from build123d import *

# Parameters (mm, degrees)
SKETCH_1_R                      = 12.55
EXTRUDE_1_DEPTH                 = 6
SKETCH_2_R                      = 3.2
CUT_EXTRUDE_1_DEPTH             = 6
CUT_EXTRUDE_2_REACH             = 20.735
SKETCH_3_R                      = 1
CUT_EXTRUDE_2_DIRECTION_2_REACH = 20.735
SKETCH_4_R                      = 13.5
EXTRUDE_2_DEPTH                 = 5
SKETCH_5_R                      = 12.5
CUT_EXTRUDE_3_DEPTH             = 5
FILLET_2_R                      = 2


with BuildPart() as part:
    # 草图1 → 凸台-拉伸1 (new body)
    with BuildSketch(Plane(origin=(0, 0, 0), x_dir=(0, 0, -1), z_dir=(1, 0, 0))):
        Circle(SKETCH_1_R)
    extrude(amount=EXTRUDE_1_DEPTH)

    # 草图2 → 切除-拉伸1 (cut)
    with BuildSketch(Plane.ZY):
        Circle(SKETCH_2_R)
    extrude(amount=-CUT_EXTRUDE_1_DEPTH, mode=Mode.SUBTRACT)

    # 草图3 → 切除-拉伸2 (cut, up to next)
    with BuildSketch(Plane(origin=(0, 0, 0), x_dir=(1, 0, 0), z_dir=(0, 1, 0)), mode=Mode.PRIVATE) as cut_extrude_2_sk1:
        with Locations(Location((3, 0, 0), (0, 0, 270))):
            Circle(SKETCH_3_R)
    cut_extrude_2_tool1 = extrude(cut_extrude_2_sk1.sketch, amount=-CUT_EXTRUDE_2_REACH, mode=Mode.PRIVATE) & part.part
    add(cut_extrude_2_tool1.solids().sort_by_distance((3, 0, 0))[0], mode=Mode.SUBTRACT)

    # 草图3 → 切除-拉伸2 direction 2 (cut, up to next)
    with BuildSketch(Plane(origin=(0, 0, 0), x_dir=(1, 0, 0), z_dir=(0, 1, 0)), mode=Mode.PRIVATE) as cut_extrude_2_direction_2_sk1:
        with Locations(Location((3, 0, 0), (0, 0, 270))):
            Circle(SKETCH_3_R)
    cut_extrude_2_direction_2_tool1 = extrude(cut_extrude_2_direction_2_sk1.sketch, amount=CUT_EXTRUDE_2_DIRECTION_2_REACH, mode=Mode.PRIVATE) & part.part
    add(cut_extrude_2_direction_2_tool1.solids().sort_by_distance((3, 0, 0))[0], mode=Mode.SUBTRACT)

    # 草图4 → 凸台-拉伸2 (add)
    with BuildSketch(Plane(origin=(6, 0, 0), x_dir=(0, 0, -1), z_dir=(1, 0, 0))):
        Circle(SKETCH_4_R)
    extrude(amount=EXTRUDE_2_DEPTH)

    # 草图5 → 切除-拉伸3 (cut)
    with BuildSketch(Plane(origin=(11, 0, 0), x_dir=(0, 0, -1), z_dir=(1, 0, 0))):
        Circle(SKETCH_5_R)
    extrude(amount=-CUT_EXTRUDE_3_DEPTH, mode=Mode.SUBTRACT)

    # 圆角2
    # the kernel refuses this fillet: 2 mm, written as the material it adds along each edge
    with BuildSketch(Plane(origin=(6, 0, 0), x_dir=(0, 0, -1), z_dir=(0, -1, 0))) as fillet_2_piece_1:
        with BuildLine():
            CenterArc((14.55, -1.702204453), FILLET_2_R, 121.668243254, 58.331756746)
            Line((12.55, -1.702204453), (12.51, -1.702204453))
            Line((12.51, -1.702204453), (12.51, 0))
            Line((12.51, 0), (12.55, 0.04))
            ThreePointArc((12.55, 0.04), (13.025, 0.04), (13.479, 0.034044089))
            Line((13.479, 0.034044089), (13.5, 0))
        make_face()
    revolve(axis=Axis((6, 0, 0), (1, 0, 0)))


solid = part.part
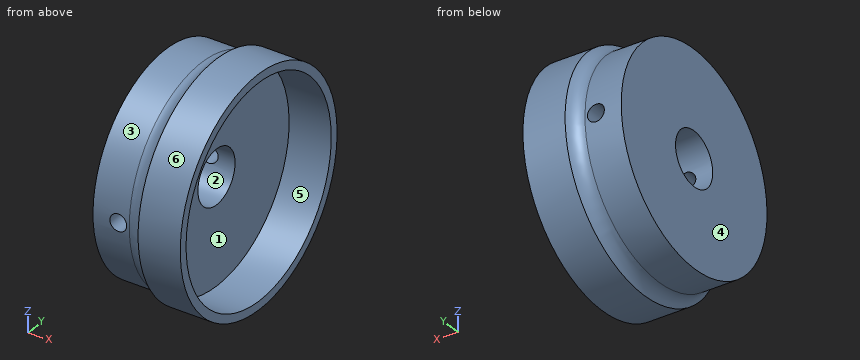
Design review of the part built by this model. Coordinates are the model's own, in mm. Face numbers are marked on the shaded views. A direction names the side the tool comes from. Give positions to 0.01 mm unless a question says otherwise; leave off trailing zeros. Order: outer loops, then holes, each group sorted by start corner. A loop starts at its lowest first (then second) coordinate and runs counter-clockwise, first axis right, second up. Notation, with made-up numbers: (16, 30.5) - (68, 30.5) arc R19 cw to (68, 53.5) - close; hole circle Ø1 at (48.25, 71.5). An arc over 180 degrees is marked (long way). Write item = value, one per line. Start each with the question number.
Q1. Tool access review of the marked faces 1, 2 and 3: name each direction out of +Z, -Z, +X, -X, +Y, -Y from which nothing blocks a thin tool from reaching the whole face with its end or side.
Q2. We need section A-A on y = 0. State the section outline as (x, z) points, plus the area to 3 significant figures.
Q3. We need section C-C on x = 3. State the section outline as (y, z) points.
Q4. We need section B-B on z = 0. State the section outline as (x, y) points.
Q5. To check wall thickness, follow L1, parallel to X at y = 7.75, z = 0; L2, parallel to X at y = 8, z = 6.5; L3, parallel to Y at x = 9.75, z = 9.75. State the ranges of each line that lie inside material, in increasing order. Write a range as from..to.
Q6. We need section D-D on x = 6.5. State the section outline as (y, z) points.
Q7. Clearance check with flat-ended pins moving along their axes: pin 1 Ø6 at (y, z) = (0, 0) entering from +X; pin 2 Ø3 at (x, z) = (2.5, -9) entering from -Y; pin 3 Ø2 at (x, z) = (2.5, -0.5) entering from +Y; pin 4 Ø3 at (x, z) = (3, 0) entering from +Y. State where each tip first meets the part, or that it passes through.
Q8. Mouldability with a two-part tool opening along Y and no side actions: class the marked faces 4, 5 and 6 as released by +Y, released by -Y, zero draft, split by the parting line, or undercut.
Working result:
q1.face_1 = +X
q1.face_2 = +X, -X
q1.face_3 = -X
q2.outline = (0, -12.55) - (4.3, -12.55) arc R2 cw to (6, -13.5) - (11, -13.5) - (11, -12.5) - (6, -12.5) - (6, -3.2) - (0, -3.2) - close; (0, 3.2) - (6, 3.2) - (6, 12.5) - (11, 12.5) - (11, 13.5) - (6, 13.5) arc R2 cw to (4.3, 12.55) - (0, 12.55) - close
q2.area = 123 mm²
q3.outline = (-12.51, -1) arc R12.55 ccw to (12.51, -1) - (3.04, -1) arc R3.2 cw to (-3.04, -1) - close; (-12.51, 1) - (-3.04, 1) arc R3.2 cw to (3.04, 1) - (12.51, 1) arc R12.55 ccw to start
q4.outline = (0, -12.55) - (2, -12.55) - (2, -3.2) - (0, -3.2) - close; (0, 3.2) - (2, 3.2) - (2, 12.55) - (0, 12.55) - close; (4, -12.55) - (4.3, -12.55) arc R2 cw to (6, -13.5) - (11, -13.5) - (11, -12.5) - (6, -12.5) - (6, -3.2) - (4, -3.2) - close; (4, 3.2) - (6, 3.2) - (6, 12.5) - (11, 12.5) - (11, 13.5) - (6, 13.5) arc R2 cw to (4.3, 12.55) - (4, 12.55) - close
q5.L1 = 0..2, 4..6
q5.L2 = 0..6
q5.L3 = -9.34..-7.82, 7.82..9.34
q6.outline = circle Ø27 at (0, 0); hole circle Ø25 at (0, 0)
q7.pin_1 = through
q7.pin_2 = -10.06
q7.pin_3 = 12.55
q7.pin_4 = 12.56
q8.face_4 = zero draft
q8.face_5 = undercut
q8.face_6 = split by the parting line
